Design review of the part shown in the three views and the two pictorial views. Dimensions are in mm from the part's minimum x, y and z. Round coordinates to 2 decimals unless told otherwise and drop trailing zeros. Order: outer loops, then holes, each group sorted by start corner. A loop starts at its lowest first (then second) coordinate and runs counter-clockwise, first axis right, second up. Notation, with made-up numbers: (31.5, -18) - (79.5, -18) arc R24 ccw to (79.5, -6) - close; hole circle Ø11 at (44.25, 7). An arc over 180 degrees is marked (long way). One line per question, with ' | ' between items. Start each with the question number.
Item 1: Add section A-A on x = 22.5. State the section outline as (y, z) points (1 decimal).
Item 2: Add section B-B on y = 12.5. State the section outline as (x, z) points, and give its area (3 significant figures).
Item 3: For L1, parallel to Z at x = 21, y = 25; L2, parallel to Y at x = 14, z = 19 (1 decimal); L3, parallel to Y at x = 3.5, z = 15.75 (1 decimal), list the stretches that pass through material, from the lowest coordinate up. Write a range as [from, to].
Item 4: Draft analysis for pull direction Y (two halves, no side actions). For the marked faces 1, 2 and 3, state which applies: +Y half, -Y half, draft (parallel to the pull), parting line (faces both ways), or undercut.
Item 5: Insertion check: pin 1 Ø1.9 at (x, z) = (27, 18.5) entering from -Y; pin 2 Ø4 at (x, y) = (5.5, 14.5) entering from +Z. Each pin has a flat end and moves straight along its axis. Give the tip position at first contact, or say it passes through.
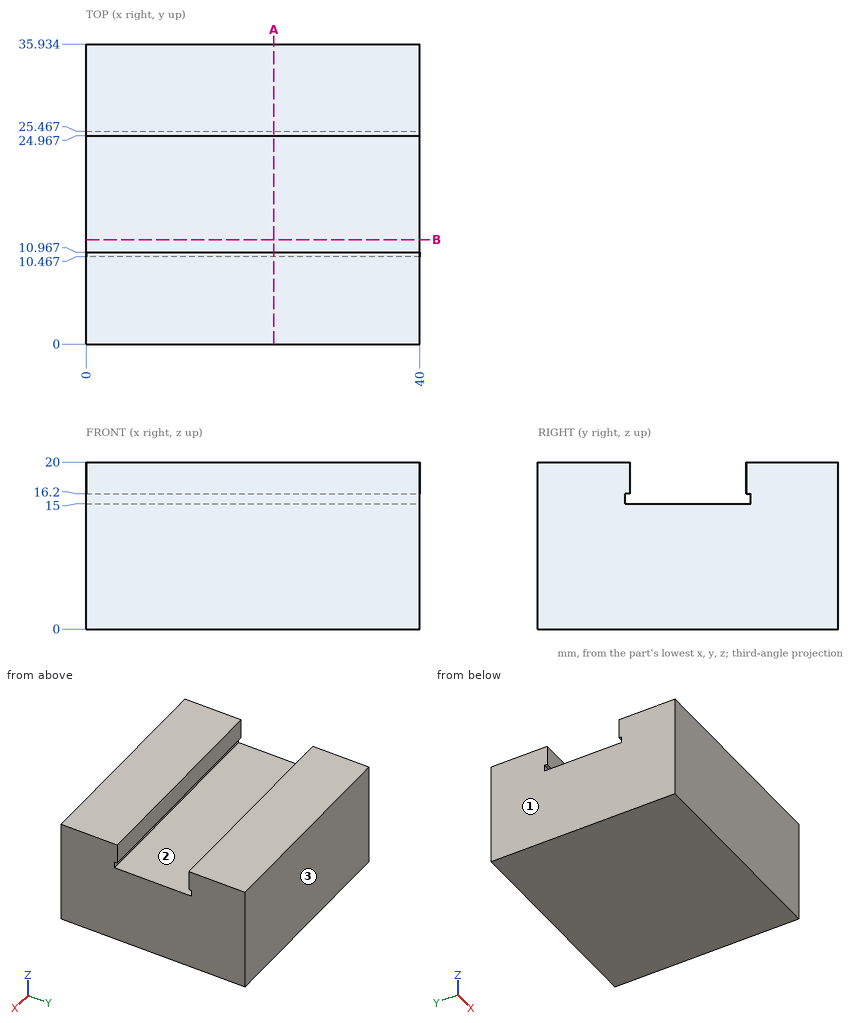
Determined:
1) outline: (0, 0) - (35.9, 0) - (35.9, 20) - (25, 20) - (25, 16.2) - (25.5, 16.2) - (25.5, 15) - (10.5, 15) - (10.5, 16.2) - (11, 16.2) - (11, 20) - (0, 20) - close
2) outline: (0, 0) - (40, 0) - (40, 15) - (0, 15) - close | area: 600 mm2
3) L1: [0, 15], [16.2, 20] | L2: [0, 11], [25, 35.9] | L3: [0, 10.5], [25.5, 35.9]
4) face 1: draft | face 2: undercut | face 3: +Y half
5) pin 1: y = 0 | pin 2: z = 15
